The model under review builds one solid part; all positions refer to its coordinate system, in mm. A direction names the side the tool comes from. Give positions to 0.01 mm unless a question says otherwise; leave off trailing zeros.
```python
from build123d import *

# Parameters (mm, degrees)
BOSS_EXTRUDE1_REACH       = 53.998
SKETCH2_R                 = 5
FILLET1_R                 = 2
M3X0_5_TAPPED_HOLE1_D     = 2.5
M3X0_5_TAPPED_HOLE1_DEPTH = 4
M3X0_5_TAPPED_HOLE1_TIP   = 0.751075774
M3X0_5_TAPPED_HOLE2_D     = 2.5
M3X0_5_TAPPED_HOLE2_DEPTH = 4
M3X0_5_TAPPED_HOLE2_TIP   = 0.751075774


with BuildPart() as part:
    # Sketch1 → Revolve1 (revolve)
    with BuildSketch(Plane.XY, mode=Mode.PRIVATE) as revolve1_sk:
        Polygon((0, 15.8), (0, -15.8), (-12.5, -15.8), (-12.5, -10.8), (-27.5, -10.8), (-27.5, -7.3), (-29.2, -7.3), (-29.2, 5.2), (-20, 8.8), (-9.5, 8.8), (-9.5, 10.8), (-2, 10.8), (-2, 15.8), align=None)
    revolve(revolve1_sk.sketch.rotate(Axis((0, 0, 0), (0, -1, 0)), 270), axis=Axis((0, 0, 0), (0, -1, 0)))

    # Sketch2 → Boss-Extrude1 (add, up to next)
    with BuildSketch(Plane.XZ.offset(15.8), mode=Mode.PRIVATE) as boss_extrude1_sk1:
        with Locations((0, 12.5)):
            Circle(SKETCH2_R)
    boss_extrude1_tool1 = extrude(boss_extrude1_sk1.sketch, amount=-BOSS_EXTRUDE1_REACH, mode=Mode.PRIVATE) - part.part
    # Sketch2 → Boss-Extrude1 (add, up to next)
    with BuildSketch(Plane.XZ.offset(15.8), mode=Mode.PRIVATE) as boss_extrude1_sk2:
        with Locations((12.5, 0)):
            Circle(SKETCH2_R)
    boss_extrude1_tool2 = extrude(boss_extrude1_sk2.sketch, amount=-BOSS_EXTRUDE1_REACH, mode=Mode.PRIVATE) - part.part
    # Sketch2 → Boss-Extrude1 (add, up to next)
    with BuildSketch(Plane.XZ.offset(15.8), mode=Mode.PRIVATE) as boss_extrude1_sk3:
        with Locations((0, -12.5)):
            Circle(SKETCH2_R)
    boss_extrude1_tool3 = extrude(boss_extrude1_sk3.sketch, amount=-BOSS_EXTRUDE1_REACH, mode=Mode.PRIVATE) - part.part
    # Sketch2 → Boss-Extrude1 (add, up to next)
    with BuildSketch(Plane.XZ.offset(15.8), mode=Mode.PRIVATE) as boss_extrude1_sk4:
        with Locations((-12.5, 0)):
            Circle(SKETCH2_R)
    boss_extrude1_tool4 = extrude(boss_extrude1_sk4.sketch, amount=-BOSS_EXTRUDE1_REACH, mode=Mode.PRIVATE) - part.part
    add(boss_extrude1_tool1.solids().sort_by_distance((0, -15.8, 12.5))[0])
    add(boss_extrude1_tool2.solids().sort_by_distance((12.5, -15.8, 0))[0])
    add(boss_extrude1_tool3.solids().sort_by_distance((0, -15.8, -12.5))[0])
    add(boss_extrude1_tool4.solids().sort_by_distance((-12.5, -15.8, 0))[0])

    # Fillet1
    fillet1_edges = [part.edges().sort_by_distance(p)[0] for p in [
        (4.898979486, -13.3, 11.5),
        (-4.898979486, -13.3, 11.5),
        (11.5, -13.3, -4.898979486),
        (11.5, -13.3, 4.898979486),
        (-4.898979486, -13.3, -11.5),
        (4.898979486, -13.3, -11.5),
        (-11.5, -13.3, 4.898979486),
        (-11.5, -13.3, -4.898979486),
    ]]
    fillet(fillet1_edges, radius=FILLET1_R)

    # M3x0.5 Tapped Hole1
    with Locations(Plane(origin=(0, -15.8, 0), x_dir=(-1, 0, 0), z_dir=(0, -1, 0))):
        with Locations((0, -12.5), (-12.5, 0), (0, 12.5), (12.5, 0)):
            Hole(M3X0_5_TAPPED_HOLE1_D / 2, depth=M3X0_5_TAPPED_HOLE1_DEPTH)
            with Locations((0, 0, -(M3X0_5_TAPPED_HOLE1_DEPTH + M3X0_5_TAPPED_HOLE1_TIP / 2))):  # 118° drill point
                Cone(0, M3X0_5_TAPPED_HOLE1_D / 2, M3X0_5_TAPPED_HOLE1_TIP, mode=Mode.SUBTRACT)

    # Sketch5 → Revolve2 (revolve)
    with BuildSketch(Plane.XY, mode=Mode.PRIVATE) as revolve2_sk:
        Polygon((0, -15.8), (-3.4, -15.8), (-3.4, -17.3), (-5.25, -17.3), (-5.25, -18.3), (-3.4, -18.3), (-3.4, -19.3), (0, -19.3), align=None)
    revolve(revolve2_sk.sketch.rotate(Axis((0, 0, 0), (0, -1, 0)), 270), axis=Axis((0, 0, 0), (0, -1, 0)))

    # M3x0.5 Tapped Hole2
    with Locations(Plane(origin=(0, 10.8, 0), x_dir=(1, 0, 0), z_dir=(0, 1, 0))):
        with Locations((0, 6), (5.196152423, 3), (5.196152423, -3), (0, -6), (-5.196152423, -3), (-5.196152423, 3)):
            Hole(M3X0_5_TAPPED_HOLE2_D / 2, depth=M3X0_5_TAPPED_HOLE2_DEPTH)
            with Locations((0, 0, -(M3X0_5_TAPPED_HOLE2_DEPTH + M3X0_5_TAPPED_HOLE2_TIP / 2))):  # 118° drill point
                Cone(0, M3X0_5_TAPPED_HOLE2_D / 2, M3X0_5_TAPPED_HOLE2_TIP, mode=Mode.SUBTRACT)


solid = part.part
```
Item 1: For line 1 (Z direction, x = 12.5, y = -12.6); line 2 (X direction, y = -14, z = 0.5); line 3 (Y direction, x = 1, z = 15), list the stretches that pass through material, from the lowest coordinate up.
Values found:
line 1: z = -5.01 to -1.25, 1.25 to 5.01
line 2: x = -17.47 to -13.65, -11.35 to 11.35, 13.65 to 17.47
line 3: y = -15.8 to 8.8
Item 2: For faces 4 (the cylindrical face through (0.27, 8.77, -4.78)), 5 (the cylindrical face through (-0.1, -13.3, -17.5)), 6 (the flat face through (26, -7.3, -11)), 7 (the flat face through (0, 15.8, 0)), list the 3-axis set-ups (+Z, -Z, +X, -X, +Y, -Y) from which the entire face can be reached by the end or side of a thin tool; tool diameter is ignored.
Values found:
face 4: +Y
face 5: -Z, -Y
face 6: -Y
face 7: +Z, -Z, +X, -X, +Y
Item 3: Draft analysis for pull direction Z (two halves, no side actions). For faces 1 (the cylindrical face through (-13.75, -13.77, -0.05)), 2 (the cylindrical face through (-8.804, -13.265, 8.874)), 3 (the flat face through (1.1, -18.3, 3.4)), state which applies: released by +Z, released by -Z, zero draft, split by the parting line, or undercut.
Values found:
face 1: undercut
face 2: released by +Z
face 3: zero draft
Item 4: Clearance check with flat-ended pins moving along their axes: pin 1 Ø3 at (y, z) = (-0.5, 16.5) entering from -X; pin 2 Ø4 at (x, z) = (-5.2, -3) entering from -Y; pin 3 Ø4 at (x, y) = (6, -8.5) entering from +Z. State where each tip first meets the part, or that it passes through.
Values found:
pin 1: stops at x = -25.05
pin 2: stops at y = -18.3
pin 3: stops at z = 28.87
